```python
from build123d import *

# Parameters (mm, degrees)
BOSS_EXTRUDE1_DEPTH     = 2
BOSS_EXTRUDE2_DEPTH     = 1
BOSS_EXTRUDE3_DEPTH     = 12
BOSS_EXTRUDE4_REACH     = 31.886
CUT_EXTRUDE1_DEPTH      = 27.734434724
CUT_EXTRUDE1_DEPTH_BACK = 27.734434724
SKETCH6_R               = 1.25
CUT_EXTRUDE2_DEPTH      = 25.948268421
CUT_EXTRUDE3_DEPTH      = 27.830693137


with BuildPart() as part:
    # Sketch1 → Boss-Extrude1 (new body)
    with BuildSketch(Plane(origin=(0, 0, 0), x_dir=(1, 0, 0), z_dir=(0, 1, 0))):
        with BuildLine():
            Line((-7.576663768, 5.7), (-19.534464968, 4.165854918))
            ThreePointArc((-19.534464968, 4.165854918), (-23.193935143, -0.225628046), (-19.084438942, -4.199151112))
            Line((-19.084438942, -4.199151112), (-7.577930804, -5.7))
            Line((-7.577930804, -5.7), (7.577930804, -5.7))
            Line((7.577930804, -5.7), (19.084438942, -4.199151112))
            ThreePointArc((19.084438942, -4.199151112), (23.2, 0), (19.084438942, 4.199151112))
            Line((19.084438942, 4.199151112), (7.577930804, 5.7))
            Line((7.577930804, 5.7), (-7.576663768, 5.7))
        make_face()
        with BuildLine():
            Line((-7.512988467, -4.7), (-19.013197102, -3.199972787))
            ThreePointArc((-19.013197102, -3.199972787), (-22.193903464, -0.197435212), (-19.407211404, 3.173984699))
            Line((-19.407211404, 3.173984699), (-7.512777295, 4.7))
            Line((-7.512777295, 4.7), (7.512988467, 4.7))
            Line((7.512988467, 4.7), (19.013197102, 3.199972787))
            ThreePointArc((19.013197102, 3.199972787), (22.2, 0), (19.013197102, -3.199972787))
            Line((19.013197102, -3.199972787), (7.512988467, -4.7))
            Line((7.512988467, -4.7), (-7.512988467, -4.7))
        make_face(mode=Mode.SUBTRACT)
    extrude(amount=BOSS_EXTRUDE1_DEPTH)

    # Sketch2 → Boss-Extrude2 (add)
    with BuildSketch(Plane(origin=(0, 2, 0), x_dir=(1, 0, 0), z_dir=(0, 1, 0))):
        with BuildLine():
            Line((7.577930804, -5.7), (19.084438942, -4.199151112))
            ThreePointArc((19.084438942, -4.199151112), (23.2, 0), (19.084438942, 4.199151112))
            Line((19.084438942, 4.199151112), (7.577930804, 5.7))
            Line((7.577930804, 5.7), (-7.576663768, 5.7))
            Line((-7.576663768, 5.7), (-19.534464968, 4.165854918))
            ThreePointArc((-19.534464968, 4.165854918), (-23.193935143, -0.225628046), (-19.084438942, -4.199151112))
            Line((-19.084438942, -4.199151112), (-7.577930804, -5.7))
            Line((-7.577930804, -5.7), (7.577930804, -5.7))
        make_face()
    extrude(amount=BOSS_EXTRUDE2_DEPTH)

    # Sketch3 → Boss-Extrude3 (add)
    with BuildSketch(Plane(origin=(0, 3, 0), x_dir=(1, 0, 0), z_dir=(0, 1, 0))):
        Polygon((-5, 0), (-5, 5), (5, 5), (5, -5), (-5, -5), align=None)
    extrude(amount=BOSS_EXTRUDE3_DEPTH)

    # Boss-Extrude4: up to this face of the body (flat: up to its plane)
    boss_extrude4_end = Plane(part.part.faces().sort_by_distance((0.000633518, 1.5, -5.7))[0])
    # Sketch4 → Boss-Extrude4 (add, up to the picked face)
    with BuildSketch(Plane.XY.offset(5.7), mode=Mode.PRIVATE) as boss_extrude4_sk1:
        with BuildLine():
            Line((-19.103038774, 3), (-7, 3))
            Line((-7, 3), (-7, 3.485357144))
            ThreePointArc((-7, 3.485357144), (-9.86131573, 3.767251876), (-12.711609357, 4.144635751))
            ThreePointArc((-12.711609357, 4.144635751), (-15.114103805, 4.934855361), (-17.117340124, 6.478704724))
            ThreePointArc((-17.117340124, 6.478704724), (-18.375058248, 6.768970937), (-19.103038774, 5.703065825))
            Line((-19.103038774, 5.703065825), (-19.103038774, 3))
        make_face()
    boss_extrude4_tool1 = split(extrude(boss_extrude4_sk1.sketch, amount=-BOSS_EXTRUDE4_REACH, mode=Mode.PRIVATE), bisect_by=boss_extrude4_end, keep=Keep.BOTH, mode=Mode.PRIVATE)
    # Sketch4 → Boss-Extrude4 (add, up to the picked face)
    with BuildSketch(Plane.XY.offset(5.7), mode=Mode.PRIVATE) as boss_extrude4_sk2:
        with BuildLine():
            Line((7, 3.485357144), (7, 3))
            Line((7, 3), (19.103038774, 3))
            Line((19.103038774, 3), (19.103038774, 5.420959691))
            ThreePointArc((19.103038774, 5.420959691), (18.322193887, 6.584407955), (16.949634957, 6.302605569))
            ThreePointArc((16.949634957, 6.302605569), (15.0061995, 4.878805237), (12.711609357, 4.144635751))
            ThreePointArc((12.711609357, 4.144635751), (9.86131573, 3.767251876), (7, 3.485357144))
        make_face()
    boss_extrude4_tool2 = split(extrude(boss_extrude4_sk2.sketch, amount=-BOSS_EXTRUDE4_REACH, mode=Mode.PRIVATE), bisect_by=boss_extrude4_end, keep=Keep.BOTH, mode=Mode.PRIVATE)
    add(boss_extrude4_tool1.solids().sort_by(Axis((-15.203187, 4.213829, 5.7), (0, 0, -1)))[0])
    add(boss_extrude4_tool2.solids().sort_by(Axis((15.148816, 4.17304, 5.7), (0, 0, -1)))[0])

    # Sketch5 → Cut-Extrude1 (cut, two sides: drawn at the far end of the back side and taken through both)
    with BuildSketch(Plane.XZ.offset(-3).offset(-CUT_EXTRUDE1_DEPTH_BACK)):
        with BuildLine():
            ThreePointArc((19.103038774, -4.198735883), (23.2, 0), (19.103038774, 4.198735883))
            Line((19.103038774, 4.198735883), (19.103038774, -4.198735883))
        make_face()
        with BuildLine():
            ThreePointArc((19.084438942, 4.199151112), (19.093739088, 4.198953796), (19.103038774, 4.198735883))
            Line((19.103038774, 4.198735883), (19.103038774, 5.7))
            Line((19.103038774, 5.7), (7.577930804, 5.7))
            Line((7.577930804, 5.7), (19.084438942, 4.199151112))
        make_face()
        with BuildLine():
            Line((19.103038774, -5.7), (19.103038774, -4.198735883))
            ThreePointArc((19.103038774, -4.198735883), (19.093739088, -4.198953796), (19.084438942, -4.199151112))
            Line((19.084438942, -4.199151112), (7.577930804, -5.7))
            Line((7.577930804, -5.7), (19.103038774, -5.7))
        make_face()
        with BuildLine():
            Line((-19.534464968, -4.165854918), (-19.103038774, -4.221205426))
            Line((-19.103038774, -4.221205426), (-19.103038774, 4.198735883))
            ThreePointArc((-19.103038774, 4.198735883), (-23.194424582, 0.216338692), (-19.534464968, -4.165854918))
        make_face()
        Polygon((-7.576663768, -5.7), (-19.103038774, -4.221205426), (-19.103038774, -5.7), align=None)
        with BuildLine():
            Line((-19.103038774, 5.7), (-19.103038774, 4.198735883))
            ThreePointArc((-19.103038774, 4.198735883), (-19.093739088, 4.198953796), (-19.084438942, 4.199151112))
            Line((-19.084438942, 4.199151112), (-7.577930804, 5.7))
            Line((-7.577930804, 5.7), (-19.103038774, 5.7))
        make_face()
    extrude(amount=CUT_EXTRUDE1_DEPTH + CUT_EXTRUDE1_DEPTH_BACK, mode=Mode.SUBTRACT)

    # Sketch6 → Cut-Extrude2 (cut, through all)
    with BuildSketch(Plane(origin=(0, 15, 0), x_dir=(1, 0, 0), z_dir=(0, 1, 0))):
        with Locations(Location((0, 0, 0), (0, 0, 270))):
            Circle(SKETCH6_R)
    extrude(amount=-CUT_EXTRUDE2_DEPTH, mode=Mode.SUBTRACT)

    # Sketch7 → Cut-Extrude3 (cut, through all)
    with BuildSketch(Plane(origin=(0, 0, -5.7), x_dir=(-1, 0, 0), z_dir=(0, 0, -1))):
        with BuildLine():
            Line((-7, 0.6), (-7, 0))
            Line((-7, 0), (7, 0))
            Line((7, 0), (7, 0.6))
            ThreePointArc((7, 0.6), (6.707106781, 1.307106781), (6, 1.6))
            Line((6, 1.6), (-6, 1.6))
            ThreePointArc((-6, 1.6), (-6.707106781, 1.307106781), (-7, 0.6))
        make_face()
    extrude(amount=-CUT_EXTRUDE3_DEPTH, mode=Mode.SUBTRACT)


solid = part.part
```
Read the model definition and answer for the solid it produces. Units are mm, in the model's axes. A direction names the side the tool comes from. Round coordinates to 2 decimals unless told otherwise and drop trailing zeros. Write each loop counter-clockwise with the first axis right and the second up, starting at its lowest first coordinate (ties: lowest second). Pieces come first, ordered by that corner, then holes. Notation, with made-up numbers: M -28.5,17 L 25.5,17 A10 cw 25.5,23 Z; hole C -0.75,46 d11. An arc over 180 degrees is marked long. One line per item, written item: value.
Q1. Flat-ended cylindrical pins translate along their axes: pin 1 Ø4 at (x, z) = (-10.5, -4) entering from +Y; pin 2 Ø8 at (x, y) = (-2, 10) entering from -Z; pin 3 Ø6 at (x, z) = (-6, -4.5) entering from -Y; pin 4 Ø6 at (x, z) = (3.5, -2.5) entering from -Y. Find the tip coordinate at first contact, or state that the pin passes through.
Data:
pin 1: y = 4.11
pin 2: z = -5
pin 3: y = 0
pin 4: y = 1.6
Q2. Find section D-D on x = 6.5. Write down the section's boundary in (y, z).
Data:
outline: M 1.47,-5.7 L 3,-5.7 L 3,5.7 L 1.47,5.7 L 1.47,4.7 L 2,4.7 L 2,-4.7 L 1.47,-4.7 Z
Q3. Which of the six approach directions +Z, -Z, +X, -X, +Y, -Y give full straight-line access (tool end or side, diameter ignored) to faces 4 (the flat face through (5, 9, 0)), 5 (the flat face through (0, 2, 2)), 6 (the cylindrical face through (-1.22, 8.59, -0.27)), 7 (the cylindrical face through (6.699, 1.315, 5.193)), 8 (the flat face through (0, 2, 5.7))?
Data:
face 4: +Z, -Z, +Y
face 5: -Y
face 6: +Y, -Y
face 7: +Z, -Z, -Y
face 8: +Z, +X, -X, +Y, -Y
Q4. Find section C-C on y = 11.25. Write down the section's boundary in (x, z), plus the area to 3 significant figures.
Data:
outline: M -5,-5 L 5,-5 L 5,5 L -5,5 Z; hole C 0,0 d2.5
area: 95.1 mm2
Q5. Straight lines are drawn through the part: line 1 (X direction, y = 6.25, z = 0); line 2 (X direction, y = 5, z = 0); line 3 (Y direction, x = -4, z = 3.25). For each, find the intervals that lie inside material, in ascending order. Write a range as [from, to].
Data:
line 1: [-18.96, -16.9], [-5, -1.25], [1.25, 5], [16.9, 18.79]
line 2: [-19.1, -15.23], [-5, -1.25], [1.25, 5], [15.23, 19.1]
line 3: [2, 15]
Q6. Find section A-A on z = 0. Write down the section's boundary in (x, y).
Data:
outline: M -19.1,2 L -1.25,2 L -1.25,15 L -5,15 L -5,3 L -7,3 L -7,3.49 A86 cw -12.71,4.14 A7.5 cw -17.12,6.48 A1.14 ccw -19.1,5.7 Z; M 1.25,2 L 19.1,2 L 19.1,5.42 A1.26 ccw 16.95,6.3 A7.5 cw 12.71,4.14 A86 cw 7,3.49 L 7,3 L 5,3 L 5,15 L 1.25,15 Z
Q7. Find section B-B on x = 0. Write down the section's boundary in (y, z).
Data:
outline: M 1.6,-5.7 L 3,-5.7 L 3,-5 L 15,-5 L 15,-1.25 L 2,-1.25 L 2,-4.7 L 1.6,-4.7 Z; M 1.6,4.7 L 2,4.7 L 2,1.25 L 15,1.25 L 15,5 L 3,5 L 3,5.7 L 1.6,5.7 Z
Q8. For a pull along Z with two mould halves and no side action, classify faces 1 (the flat face through (-14.69, 2.615, 4.772)), 2 (the flat face through (13.34, 0.99, 3.94)), 3 (the cylindrical face through (6.699, 1.315, -5.207)) as +Z half, -Z half, draft (parallel to the pull), parting line (faces both ways), or undercut.
Data:
face 1: +Z half
face 2: undercut
face 3: draft
